```python
from build123d import *

# Parameters (mm, degrees)
F0_W      = 132.08
F0_H      = 106.68
F0_W_2    = 127
F0_H_2    = 101.6
F1_DEPTH  = 25.4
F2_W      = 127
F2_H      = 2.0145024173
F3_DEPTH  = 101.6
F5_D      = 6.35
F2_H_2    = 2.122098887
F6_DEPTH  = 101.6
F7_W      = 82.3423601687
F7_H      = 69.9707251042
F7_W_2    = 76.2
F7_H_2    = 63.5
F8_DEPTH  = 25.4
F10_D     = 6.35
F10_DEPTH = 12.7
F10_TIP   = 1.9077324654
F11_T     = -2.54


with BuildPart() as f1:
    # F0 (on Top) → F1 (new body)
    with BuildSketch(Plane.XY):
        with Locations((4.9622115278, -0.4122621453)):
            Rectangle(F0_W, F0_H)
        with Locations((4.3762922287, -0.5259333495)):
            Rectangle(F0_W_2, F0_H_2, mode=Mode.SUBTRACT)
    extrude(amount=F1_DEPTH)

    # F2 (on face) → F3 (join)
    with BuildSketch(Plane.XZ.offset(-50.2740666505)):
        with Locations((4.3762922287, 1.0072512086)):
            Rectangle(F2_W, F2_H)
    extrude(amount=F3_DEPTH)

    # F5 (through all)
    with Locations(Plane.XZ.offset(53.7522621453)):
        with Locations((0, 11.9956443086)):
            Hole(F5_D / 2)

    # F2 (on face) → F6 (join)
    with BuildSketch(Plane.XZ.offset(-50.2740666505)):
        with Locations((4.3762922287, 24.3389505565)):
            Rectangle(F2_W, F2_H_2)
        with Locations((4.3762922287, 1.0072512086)):
            Rectangle(F2_W, F2_H)
    extrude(amount=F6_DEPTH)

    # F7 (on face) → F8 (join)
    with BuildSketch(Plane.XY.offset(25.4)):
        with Locations((-1.2168828398, 4.8675285652)):
            Rectangle(F7_W, F7_H)
        with Locations((-1.7157470335, 5.1717488095)):
            Rectangle(F7_W_2, F7_H_2, mode=Mode.SUBTRACT)
        with Locations((-1.7157470335, 5.1717488095)):
            Rectangle(F7_W_2, F7_H_2)
    extrude(amount=F8_DEPTH)

    # F10
    with Locations(Plane.XY.offset(25.4)):
        with Locations((48.7300269306, -23.8934792578), (48.7300269306, 12.2345555574)):
            Hole(F10_D / 2, depth=F10_DEPTH)
            with Locations((0, 0, -(F10_DEPTH + F10_TIP / 2))):  # 118° drill point
                Cone(0, F10_D / 2, F10_TIP, mode=Mode.SUBTRACT)

    # F11
    f11_openings = [f1.faces().sort_by_distance(p)[0] for p in [
        (-1.216883, 4.867529, 50.8),
    ]]
    offset(amount=F11_T, openings=f11_openings)


solid = f1.part
```
CAD build for the part. Positions are in the model's coordinates, mm. A direction names the side the tool comes from. Round coordinates to 2 decimals unless told otherwise and drop trailing zeros. Write each loop counter-clockwise with the first axis right and the second up, starting at its lowest first coordinate (ties: lowest second). Pieces come first, ordered by that corner, then holes. Notation, with made-up numbers: M -35.75,88 L 18.25,88 A33 ccw 18.25,119 Z; hole C 18.25,75.5 d2. An arc over 180 degrees is marked long. One line per question, with ' | ' between items.
1. Pin check, flat tips, straight feed: pin 1 Ø12.5 at (x, z) = (8.5, 37) entering from +Y; pin 2 Ø8 at (x, y) = (46, 35) entering from +Z; pin 3 Ø8.5 at (x, z) = (0, 12) entering from -Y; pin 4 Ø2 at (x, y) = (34.5, -11) entering from +Z. Stop position of each tip, or through.
Working result:
pin 1: y = 39.85 | pin 2: z = 25.4 | pin 3: y = -53.75 | pin 4: z = 25.82
2. Cut at B-B on y = 46. Write the cut outline in (x, z), and give its area (3 significant figures).
Working result:
outline: M -61.08,0 L 71,0 L 71,25.4 L -61.08,25.4 Z; hole M -59.12,2.01 L 67.88,2.01 L 67.88,23.28 L -59.12,23.28 Z | area: 654 mm2
3. Cut at A-A on x = 0. Write the cut outline in (y, z).
Working result:
outline: M -53.75,0 L 52.93,0 L 52.93,8.82 L 50.27,8.82 L 50.27,2.01 L -51.33,2.01 L -51.33,8.82 L -53.75,8.82 Z; M -53.75,15.17 L -51.33,15.17 L -51.33,23.28 L 50.27,23.28 L 50.27,15.17 L 52.93,15.17 L 52.93,25.4 L 39.85,25.4 L 39.85,50.8 L 37.31,50.8 L 37.31,25.82 L -27.58,25.82 L -27.58,50.8 L -30.12,50.8 L -30.12,25.4 L -53.75,25.4 Z
4. Which spindle directions (+Z, -Z, +X, -X, +Y, -Y) get a long thin tool onto all of the face, cutting with end or side? Do faces 4 (the flat face through (-59.124, -1, 12)), 5 (the cylindrical face through (51.9, -23.75, 24.32)), 6 (the flat face through (-2, 39.853, 38)), 7 (the flat face through (39.954, 4, 38)). Say none if no direction does.
Working result:
face 4: none | face 5: +Z | face 6: +Z, +X, -X, +Y | face 7: +Z, +X, +Y, -Y
5. Cut at C-C on x = 20. Write the cut outline in (y, z), and give its area (3 significant figures).
Working result:
outline: M -53.75,0 L 52.93,0 L 52.93,25.4 L 39.85,25.4 L 39.85,50.8 L 37.31,50.8 L 37.31,25.82 L -27.58,25.82 L -27.58,50.8 L -30.12,50.8 L -30.12,25.4 L -53.75,25.4 Z; hole M -51.33,2.01 L 50.27,2.01 L 50.27,23.28 L -51.33,23.28 Z | area: 705 mm2
6. Mould opens along Y. For faces 1 (the cylindrical face through (-3.03, 51.62, 12.95)), 2 (the flat face through (3.5, 50.274, 12.5)), 3 (the flat face through (4, 52.928, 13)) say: pulls with the +Y half, pulls with the -Y half, needs draft (parallel to the pull), parting line crosses it, or undercut.
Working result:
face 1: needs draft | face 2: undercut | face 3: pulls with the +Y half
7. Probe L1, parallel to Z at x = 18.5, y = 43.5; L2, parallel to Y at x = 29, z = 17; L3, parallel to Y at x = -6, z = 43.5. List the from-to ranges inside material, lowest first. Write a range as from..to.
Working result:
L1: 0..2.01, 23.28..25.4 | L2: -53.75..-51.33, 50.27..52.93 | L3: -30.12..-27.58, 37.31..39.85
8. Cut at D-D on y = 26. Write the cut outline in (x, z), and give its area (3 significant figures).
Working result:
outline: M -61.08,0 L 71,0 L 71,25.4 L 39.95,25.4 L 39.95,50.8 L 37.41,50.8 L 37.41,25.82 L -39.85,25.82 L -39.85,50.8 L -42.39,50.8 L -42.39,25.4 L -61.08,25.4 Z; hole M -59.12,2.01 L 67.88,2.01 L 67.88,23.28 L -59.12,23.28 Z | area: 816 mm2
